Geometry: final body of the model. Coordinates: model frame, mm. A direction names the side the tool comes from. Coordinates: 2 decimals unless noted, no trailing zeros. Write each loop counter-clockwise with the first axis right and the second up, starting at its lowest first coordinate (ties: lowest second). Pieces come first, ordered by that corner, then holes. Notation, with made-up numbers: (12, 27.25) - (25, 27.25) arc R19 ccw to (25, 41.25) - close; hole circle Ø7 at (40.5, 72). An arc over 180 degrees is marked (long way). Put each result on its own line as item: value.
```python
from build123d import *

# Parameters (mm, degrees)
F0_R        = 9.525
F1_DEPTH    = 6.35
F2_W        = 12.7
F2_H        = 6.35
F3_DEPTH    = 9.525
F4_R        = 10.922
F5_DEPTH    = 2.54
F6_W        = 25.4
F6_H        = 5.588
F7_DEPTH    = 9.525
F8_R        = 5.08
F9_T1_DEPTH = 30.7887812379
F10_R       = 6.35
F11_R       = 1.905
F12_DEPTH   = 13.336


# Not quite as in the source:
# - a fillet or chamfer that OpenCascade refuses, or shapes differently, is made with other operations: its cross-section is extruded or revolved along the edge and cut away or added


with BuildPart() as f1:
    # F0 (on Front) → F1 (new body)
    with BuildSketch(Plane.XZ):
        Circle(F0_R)
    extrude(amount=F1_DEPTH)

    # F2 (on face) → F3 (join)
    with BuildSketch(Plane(origin=(0, 0, 0), x_dir=(-1, 0, 0), z_dir=(0, 1, 0))):
        Rectangle(F2_W, F2_H)
    extrude(amount=F3_DEPTH)

    # F4 (on face) → F5 (join)
    with BuildSketch(Plane.XZ.offset(6.35)):
        Circle(F4_R)
    extrude(amount=F5_DEPTH)

    # F6 (on face) → F7 (join)
    with BuildSketch(Plane.XZ.offset(8.89)):
        with Locations((-10.922, -0.381)):
            Rectangle(F6_W, F6_H)
    extrude(amount=F7_DEPTH)

    # F8
    f8_edges = [f1.edges().sort_by_distance(p)[0] for p in [
        (-23.622, -18.415, -0.381),
    ]]
    fillet(f8_edges, radius=F8_R)

    # F9: fillet of radius 5.08 on 1 edges, made by hand

    # F9_s2 → F9_t1 (cut)
    with BuildSketch(Plane.XY.offset(-15.7753906189)):
        with BuildLine():
            ThreePointArc((-23.622, -13.335), (-21.9419479175, -10.16), (-18.5818437524, -8.89))
            Line((-18.5818437524, -8.89), (-23.622, -8.89))
            Line((-23.622, -8.89), (-23.622, -13.335))
        make_face()
    extrude(amount=F9_T1_DEPTH, mode=Mode.SUBTRACT)

    # F10
    f10_edges = [f1.edges().sort_by_distance(p)[0] for p in [
        (1.778, -18.415, -0.381),
    ]]
    fillet(f10_edges, radius=F10_R)

    # F11 (on face) → F12 (cut, through all)
    with BuildSketch(Plane.XY.offset(2.413)):
        with Locations((-19.05, -13.6525)):
            Circle(F11_R)
    extrude(amount=-F12_DEPTH, mode=Mode.SUBTRACT)


solid = f1.part
```
1. Section query D-D (x = 3). Return loops of the section in (y, z) (3 decimals).
Answer below:
outline: (-8.89, -10.502) - (-6.35, -10.502) - (-6.35, -9.04) - (0, -9.04) - (0, -3.175) - (9.525, -3.175) - (9.525, 3.175) - (0, 3.175) - (0, 9.04) - (-6.35, 9.04) - (-6.35, 10.502) - (-8.89, 10.502) - close
2. Section query A-A (x = -19.05). Return loops of the section in (y, z) (1 decimal), then the cut area to 3 significant figures.
Answer below:
outline: (-18.4, -3.2) - (-15.6, -3.2) - (-15.6, 2.4) - (-18.4, 2.4) - close; (-11.7, -3.2) - (-8.9, -3.2) - (-8.9, 2.4) - (-11.7, 2.4) - close
area: 31.7 mm²
3. Section query C-C (y = 3.25). Return loops of the section in (x, z) (3 decimals), then the cut area to 3 significant figures.
Answer below:
outline: (-6.35, -3.175) - (6.35, -3.175) - (6.35, 3.175) - (-6.35, 3.175) - close
area: 80.6 mm²
4. Section query B-B (z = -5.25). Return loops of the section in (x, y), then the cut area to 3 significant figures.
Answer below:
outline: (-9.58, -8.89) - (9.58, -8.89) - (9.58, -6.35) - (7.95, -6.35) - (7.95, 0) - (-7.95, 0) - (-7.95, -6.35) - (-9.58, -6.35) - close
area: 150 mm²
5. Mould query, pull axis X, two halves, no side actions, for faces 1 (the cylindrical face through (10.418, -7.602, 3.281)), 2 (the cylindrical face through (-17.233, -13.08, -0.342)), 3 (the flat face through (6.35, 5, 0)). Classes: +X half, -X half, draft (parallel to the pull), parting line (faces both ways), or undercut.
Answer below:
face 1: parting line
face 2: undercut
face 3: +X half
6. Ray query, probe 1 along X at (y, z) = (4.5, 2.5); probe 2 along Y at (x, z) = (-7, 0.75) (3 decimals); probe 3 along Y at (x, z) = (4, -2.5) (3 decimals). Return the intervals inside material, ascending. Write a range as from..to.
Answer below:
probe 1: x = -6.35..6.35
probe 2: y = -18.415..0
probe 3: y = -8.89..9.525
7. Set-up query: faces 4 (the flat face through (-6.35, 5, 0)), 5 (the flat face through (0, 5, 3.175)), 6 (the flat face through (-11, -14, -3.175)), 7 (the flat face through (-11, -14, 2.413)), 8 (the cylindrical face through (-7.559, -3.131, -5.796)). Return all of +Z, -Z, +X, -X, +Y, -Y with unobstructed straight access to the full face (end or side cutting, diameter ignored); none if empty.
Answer below:
face 4: +Z, -Z, -X, +Y
face 5: +Z, +X, -X, +Y
face 6: -Z, +X, -X, -Y
face 7: +Z, +X, -X, -Y
face 8: +Y
8. Pin query (flat end, axial travel): pin 1 Ø5 at (x, y) = (-16.5, -15) entering from -Z (3 decimals); pin 2 Ø10.5 at (x, y) = (-3, 5) entering from +Z; pin 3 Ø4.5 at (x, z) = (-15, -1.5) entering from +Y; pin 4 Ø5 at (x, y) = (0, -10.5) entering from +Z. Return the tip coordinate at first contact, or that it passes through.
Answer below:
pin 1: stops at z = -3.175
pin 2: stops at z = 9.42
pin 3: stops at y = -8.89
pin 4: stops at z = 10.92
